```python
from build123d import *

# Parameters (mm, degrees)
BOSS_EXTRUDE1_DEPTH = 123.83
FILLET1_R           = 3.175


with BuildPart() as part:
    # Sketch1 → Boss-Extrude1 (new body, symmetric)
    with BuildSketch(Plane.XY):
        Polygon((0, 25.4), (0, 0), (25.4, 0), (25.4, 3.175), (3.175, 3.175), (3.175, 25.4), align=None)
    extrude(amount=BOSS_EXTRUDE1_DEPTH, both=True)

    # Fillet1
    fillet1_edges = [part.edges().sort_by_distance(p)[0] for p in [
        (3.175, 3.175, 0),
    ]]
    fillet(fillet1_edges, radius=FILLET1_R)


solid = part.part
```
Model file for the job. Use its own axes, mm. A direction names the side the tool comes from. Coordinates: 2 decimals unless noted, no trailing zeros. Order: outer loops, then holes, each group sorted by start corner. A loop starts at its lowest first (then second) coordinate and runs counter-clockwise, first axis right, second up. Notation, with made-up numbers: M 0,-24.5 L 10,-24.5 A18 ccw 10,9.5 Z; hole C 62,-16.75 d7. An arc over 180 degrees is marked long. Answer as CSV lines item,"result".
(1) Flat gauge pins, fed straight in: pin 1 (9.5 mm diameter, centred on y = 12, z = -29.5, fed in from +X) (3 decimals); pin 2 (3 mm diameter, centred on x = 10, z = 32, fed in from -Y); pin 3 (3 mm diameter, centred on x = 7, z = 70, fed in from +Y); pin 4 (9.5 mm diameter, centred on x = 19.5, z = -51.5, fed in from +Y) (3 decimals). Where does each tip first touch, or does it go through?
Geometry says:
pin 1,"stops at x = 3.175"
pin 2,"stops at y = 0"
pin 3,"stops at y = 3.29"
pin 4,"stops at y = 3.175"
(2) Band-saw the part on A-A, the plane z = -39.5. List the corners of the cut face in (x, y) (3 decimals), then the cut area to 3 significant figures.
Geometry says:
outline,"M 0,0 L 25.4,0 L 25.4,3.175 L 6.35,3.175 A3.175 cw 3.175,6.35 L 3.175,25.4 L 0,25.4 Z"
area,"153 mm2"
(3) 3-axis set-ups, long thin cutter, end or side, ignore diameter. For faces 1 (the flat face through (3, 5, 123.83)), 2 (the flat face through (3.175, 16, 2)): which of +Z, -Z, +X, -X, +Y, -Y reach the whole face in a straight line?
Geometry says:
face 1,"+Z, +X, -X, +Y, -Y"
face 2,"+Z, -Z, +X, +Y"
(4) Wall check: line 1 along X through (y, z) = (13.75, 54) (3 decimals); line 2 along Y through (x, z) = (3.5, 12). Give the ranges that are in metal, low to high.
Geometry says:
line 1,"x = 0 to 3.175"
line 2,"y = 0 to 4.95"
(5) Band-saw the part on B-B, the plane x = 15.75. List the corners of the cut face in (y, z) (3 decimals).
Geometry says:
outline,"M 0,-123.83 L 3.175,-123.83 L 3.175,123.83 L 0,123.83 Z"
